Check sheet for the modelled part. Datum: model origin and axes. Units: mm. A direction names the side the tool comes from. Round coordinates to 2 decimals unless told otherwise and drop trailing zeros. Write each loop counter-clockwise with the first axis right and the second up, starting at its lowest first coordinate (ties: lowest second). Pieces come first, ordered by that corner, then holes.
Item 1: Go/stop test with a flat-tipped pin: pin 1 Ø6.5 at (x, y) = (168.5, 430.5) entering from -Z (3 decimals). Record where the tip stops, or that it passes through.
Item 2: Cross-section at A-A on y = 425.45. Enter the section's corners in (x, z) (3 decimals), plus the area to 3 significant figures.
Item 3: Material ranges on line 1 (Y direction, x = 181, z = 9); line 2 (X direction, y = 425.45, z = 9.5) (3 decimals), recorded low to high.
Item 4: Release check for a two-part mould opening along X. For faces 1 (the flat face through (203.2, 269, 9)), 2 (the flat face through (0, 269, 9)), 3 (the flat face through (100, 277, 19.05)), 4 (the flat face through (163.5, 420.7, 6.985)) record: +X half, -X half, draft (parallel to the pull), parting line (faces both ways), or undercut.
Item 5: Tool access check on faces 5 (the flat face through (100, 0, 9)), 6 (the cylindrical face through (176.381, 432.883, 3.444)). Record the directions out of +Z, -Z, +X, -X, +Y, -Y that give a thin tool (end or side, any length) a straight path to the whole face; none if there is none.
Item 6: Cross-section at B-B on y = 495.3. Enter the section's corners in (x, z).
from build123d import *

# Parameters (mm, degrees)
SKETCH1_W               = 203.2
SKETCH1_H               = 546.1
BOSS_EXTRUDE1_DEPTH     = 19.05
SKETCH2_R               = 19.2405
CUT_EXTRUDE1_DEPTH      = 583.990868282
ESQUISSE1_R             = 10.9982
ENL_V_MAT_EXTRU_1_DEPTH = 6.985
ESQUISSE2_R             = 6.35
ENL_V_MAT_EXTRU_2_DEPTH = 583.804439092


with BuildPart() as part:
    # Sketch1 → Boss-Extrude1 (new body)
    with BuildSketch(Plane.XY):
        with Locations((101.6, 273.05)):
            Rectangle(SKETCH1_W, SKETCH1_H)
    extrude(amount=BOSS_EXTRUDE1_DEPTH)

    # Sketch2 → Cut-Extrude1 (cut, through all)
    with BuildSketch(Plane(origin=(0, 0, 0), x_dir=(-1, 0, 0), z_dir=(0, 0, -1))):
        with Locations((-168.275, 495.3)):
            Circle(SKETCH2_R)
        with Locations((-168.275, 355.6)):
            Circle(SKETCH2_R)
    extrude(amount=-CUT_EXTRUDE1_DEPTH, mode=Mode.SUBTRACT)

    # Esquisse1 → Enlèv. mat.-Extru.1 (cut)
    with BuildSketch(Plane(origin=(0, 0, 0), x_dir=(-1, 0, 0), z_dir=(0, 0, -1))):
        with Locations((-168.275, 425.45)):
            Circle(ESQUISSE1_R)
    extrude(amount=-ENL_V_MAT_EXTRU_1_DEPTH, mode=Mode.SUBTRACT)

    # Esquisse2 → Enlèv. mat.-Extru.2 (cut, through all)
    with BuildSketch(Plane(origin=(0, 0, 6.985), x_dir=(-1, 0, 0), z_dir=(0, 0, -1))):
        with Locations((-168.275, 425.45)):
            Circle(ESQUISSE2_R)
    extrude(amount=-ENL_V_MAT_EXTRU_2_DEPTH, mode=Mode.SUBTRACT)


solid = part.part
Response values:
1. pin 1: stops at z = 6.985
2. outline: (0, 0) - (157.277, 0) - (157.277, 6.985) - (161.925, 6.985) - (161.925, 19.05) - (0, 19.05) - close; (174.625, 6.985) - (179.273, 6.985) - (179.273, 0) - (203.2, 0) - (203.2, 19.05) - (174.625, 19.05) - close
2. area: 3,560 mm2
3. line 1: y = 0 to 341.17, 370.03 to 480.87, 509.73 to 546.1
3. line 2: x = 0 to 161.925, 174.625 to 203.2
4. face 1: +X half
4. face 2: -X half
4. face 3: draft
4. face 4: undercut
5. face 5: +Z, -Z, +X, -X, -Y
5. face 6: -Z
6. outline: (0, 0) - (149.03, 0) - (149.03, 19.05) - (0, 19.05) - close; (187.52, 0) - (203.2, 0) - (203.2, 19.05) - (187.52, 19.05) - close
